The model under review builds one solid part; all positions refer to its coordinate system, in mm. A direction names the side the tool comes from. Coordinates: 2 decimals unless noted, no trailing zeros. Order: outer loops, then holes, each group sorted by start corner. A loop starts at its lowest first (then second) coordinate and runs counter-clockwise, first axis right, second up. Notation, with made-up numbers: (-11, 9.25) - (11, 9.25) arc R33 ccw to (11, 40.25) - close; hole circle Ø4 at (76, 18.25). An arc over 180 degrees is marked (long way). Answer in a Markdown table with one row per item.
Autodesk Inventor part; units mm, degrees
ref_plane "YZ Plane" through (0, 0, 0) normal (1, 0, 0) x (0, 1, 0)
ref_plane "XZ Plane" through (0, 0, 0) normal (0, 1, 0) x (-1, 0, 0)
ref_plane "XY Plane" through (0, 0, 0) normal (0, 0, 1) x (1, 0, 0)
sketch "Sketch1" plane through (0, 0, 0) normal (0, 0, 1) x (1, 0, 0)
  line L0 (0, 0) -> (58, 0)
  line L1 (58, 0) -> (58, 8)
  line L2 (58, 8) -> (0, 8)
  line L3 (0, 8) -> (0, 0)
  circle A0 centre (0, 2) radius 6
  circle A1 centre (58, 2) radius 6
  dimension "d88" = 12
  dimension "d0" = 58
  dimension "d1" = 8
extrude "Extrusion1" add sketch "Sketch1" along normal blind 3
fillet "圓角5" radius 5 2 edges at (5.6569, 0, 1.5) (52.3431, 0, 1.5)
sketch "草圖9" plane through (0, 0, 3) normal (0, 0, 1) x (1, 0, 0)
  line L0 (0, 8) -> (58, 8)
  arc A0 (0, 8) -> (4.6283, -1.8182) centre (0, 2) ccw
  point P0 (0, 0)
  point P1 (6, 4)
  point P2 (52, 4)
  dimension "d90" = 4
  dimension "d91" = 46
  dimension "d92" = 6
hole "孔5" at (6, 4, 3) at (52, 4, 3) direction (0, 0, -1) diameter 3 end through all
properties part number "plastic_part_53"
Item 1: We need section A-A, the plane x = 52. Write out the cut boundary in (y, z).
Check values:
| item | result |
|---|---|
| outline | (-0.66, 0) - (2.5, 0) - (2.5, 3) - (-0.66, 3) - close; (5.5, 0) - (8, 0) - (8, 3) - (5.5, 3) - close |
Item 2: We need section D-D, the plane x = 39. Write out the cut boundary in (y, z).
Check values:
| item | result |
|---|---|
| outline | (0, 0) - (8, 0) - (8, 3) - (0, 3) - close |
Item 3: Mouldability with a two-part tool opening along Y and no side actions: class faces 3 (the face through (29, 3, 3)), 4 (the face through (53.464, 4.325, 1.479)), 5 (the face through (51.67, -0.49, 1.52)) as +Y half, -Y half, draft (parallel to the pull), parting line (faces both ways), or undercut.
Check values:
| item | result |
|---|---|
| face 3 | draft |
| face 4 | undercut |
| face 5 | -Y half |
Item 4: We need section B-B, the plane z = 2.3. Write out the cut boundary in (x, y).
Check values:
| item | result |
|---|---|
| outline | (0, 8) arc R6 ccw (long way) to (4.63, -1.82) arc R5 cw to (8.49, 0) - (49.51, 0) arc R5 cw to (53.37, -1.82) arc R6 ccw (long way) to (58, 8) - close; hole circle Ø3 at (6, 4); hole circle Ø3 at (52, 4) |
Item 5: To check wall thickness, follow line 1 (X direction, y = 3.5, z = 1.75); line 2 (X direction, y = 4, z = 0.8); line 3 (Y direction, x = 18, z = 1.1). State the ranges of each line that lie inside material, in increasing order. Write a range as from..to.
Check values:
| item | result |
|---|---|
| line 1 | -5.81..4.59, 7.41..50.59, 53.41..63.81 |
| line 2 | -5.66..4.5, 7.5..50.5, 53.5..63.66 |
| line 3 | 0..8 |
Item 6: Tool access review of faces 1 (the face through (29, 0, 1)), 2 (the face through (6.575, 2.614, 1.479)): name each direction out of +Z, -Z, +X, -X, +Y, -Y from which nothing blocks a thin tool from reaching the whole face with its end or side.
Check values:
| item | result |
|---|---|
| face 1 | +Z, -Z, -Y |
| face 2 | +Z, -Z |
Item 7: We need section C-C, the plane y = 4. Write out the cut boundary in (x, z).
Check values:
| item | result |
|---|---|
| outline | (-5.66, 0) - (4.5, 0) - (4.5, 3) - (-5.66, 3) - close; (7.5, 0) - (50.5, 0) - (50.5, 3) - (7.5, 3) - close; (53.5, 0) - (63.66, 0) - (63.66, 3) - (53.5, 3) - close |
